The drawing under review shows one solid part. Ordinate dimensions are in mm from its lowest x, y, z. A direction names the side the tool comes from. Coordinates: 2 decimals unless noted, no trailing zeros. Order: outer loops, then holes, each group sorted by start corner. A loop starts at its lowest first (then second) coordinate and runs counter-clockwise, first axis right, second up. Notation, with made-up numbers: (-36.5, 17) - (17.5, 17) arc R29 ccw to (17.5, 49) - close; hole circle Ø5 at (57, -2). An arc over 180 degrees is marked (long way). Write item = value, one per line. Start each with the question number.
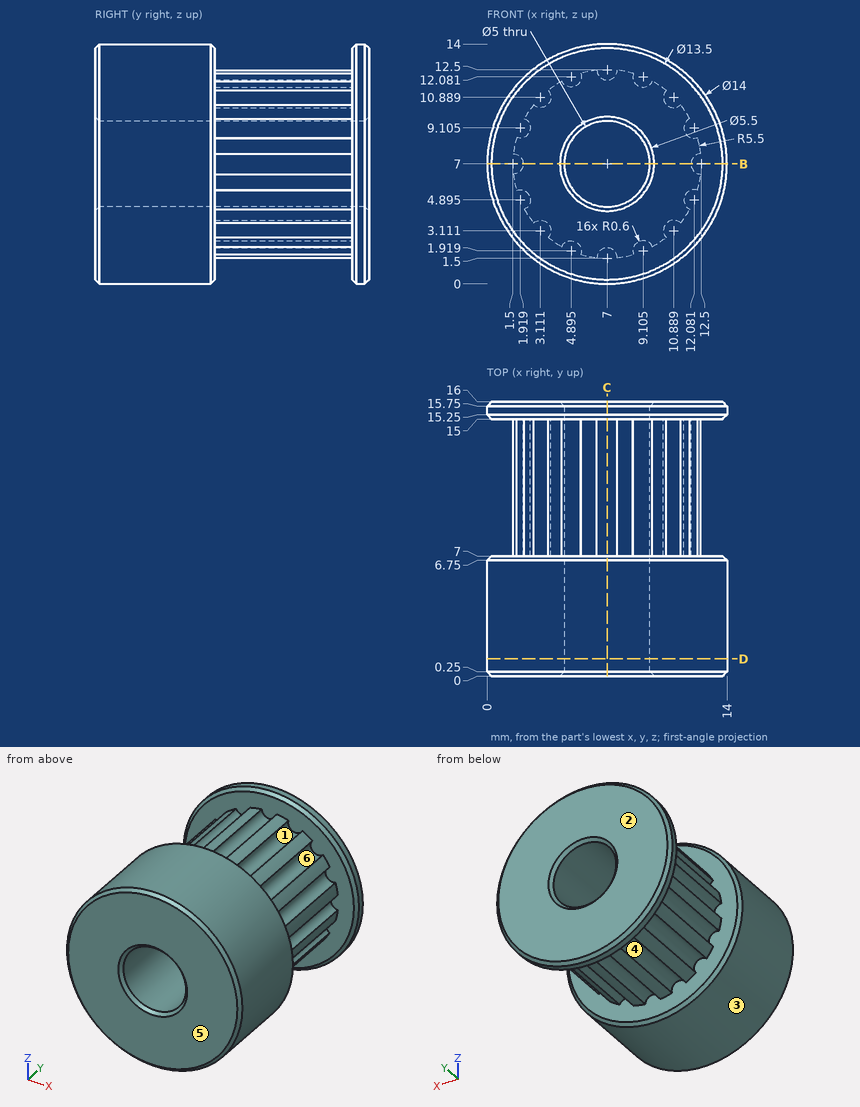
Item 1: Add section D-D on y = 1. Give the boundary of the cut face in (x, z), plus the area to 3 significant figures.
Item 2: For P1, Ø6, axis at y = 6, z = 12.5, coming from the -X side; P2, Ø3, axis at y = 7, z = 10, coming from the +X side; P3, Ø4, axis at x = 11.5, y = 7.5, coming from the +Z side, all flat-tipped, find the tip position at first contact; note any pin that passes through.
Item 3: Add section B-B on z = 7. Give the boundary of the cut face in (x, y), plus the area to 3 significant figures.
Item 4: For line 1 (Y direction, x = 9, z = 1); line 2 (Z direction, x = 7, y = 6); line 3 (Z direction, x = 7, y = 8.5), list the stretches that pass through material, from the lowest coordinate up.
Item 5: Mouldability with a two-part tool opening along Z and no side actions: class the marked faces 1, 2, 3 and 4 as +Z half, -Z half, draft (parallel to the pull), parting line (faces both ways), or undercut.
Item 6: For the marked faces 5 and 6, list the 3-axis set-ups (+Z, -Z, +X, -X, +Y, -Y) from which the entire face can be reached by the end or side of a thin tool; tool diameter is ignored.
Item 7: Add section C-C on x = 7. Give the boundary of the cut face in (y, z), plus the area to 3 significant figures.
Worked out:
q1.outline = circle Ø14 at (7, 7); hole circle Ø5 at (7, 7)
q1.area = 134 mm2
q2.P1 = 0.46
q2.P2 = 13.83
q2.P3 = 13.48
q3.outline = (0, 0.25) - (0.25, 0) - (4.25, 0) - (4.5, 0.25) - (4.5, 15.75) - (4.25, 16) - (0.25, 16) - (0, 15.75) - (0, 15.25) - (0.25, 15) - (2.1, 15) - (2.1, 7) - (0.25, 7) - (0, 6.75) - close; (9.5, 0.25) - (9.75, 0) - (13.75, 0) - (14, 0.25) - (14, 6.75) - (13.75, 7) - (11.9, 7) - (11.9, 15) - (13.75, 15) - (14, 15.25) - (14, 15.75) - (13.75, 16) - (9.75, 16) - (9.5, 15.75) - close
q3.area = 110 mm2
q4.line_1 = 0 to 7, 15 to 16
q4.line_2 = 0 to 4.5, 9.5 to 14
q4.line_3 = 2.1 to 4.5, 9.5 to 11.9
q5.face_1 = undercut
q5.face_2 = draft
q5.face_3 = parting line
q5.face_4 = undercut
q6.face_5 = +Z, -Z, +X, -X, -Y
q6.face_6 = none
q7.outline = (0, 0.25) - (0.25, 0) - (6.75, 0) - (7, 0.25) - (7, 2.1) - (15, 2.1) - (15, 0.25) - (15.25, 0) - (15.75, 0) - (16, 0.25) - (16, 4.25) - (15.75, 4.5) - (0.25, 4.5) - (0, 4.25) - close; (0, 9.75) - (0.25, 9.5) - (15.75, 9.5) - (16, 9.75) - (16, 13.75) - (15.75, 14) - (15.25, 14) - (15, 13.75) - (15, 11.9) - (7, 11.9) - (7, 13.75) - (6.75, 14) - (0.25, 14) - (0, 13.75) - close
q7.area = 110 mm2
